from build123d import *

# Parameters (mm, degrees)
EXTRUDE_1_DEPTH          = 3
EXTRUDE_START            = 58
EXTRUDE_2_DEPTH          = 58
EXTRUDE_3_DEPTH          = 0.0001
EXTRUDE_3_DEPTH_BACK     = 6
SKETCH_3_R               = 40
CUT_EXTRUDE_1_DEPTH      = 295.262309003
CUT_EXTRUDE_1_DEPTH_BACK = 295.262309003
EXTRUDE_4_REACH          = 329.042
EXTRUDE_4_END_RADIUS     = 40
SKETCH_5_R               = 28
SKETCH_5_R_2             = 24
RIB_5_REACH              = 296.262
SKETCH_9_WALL_W          = 606.033549296
SKETCH_9_WALL_H          = 6
PATTERN_CIRCULAR_1_COUNT = 4
SKETCH_10_R              = 10
CUT_EXTRUDE_2_DEPTH      = 333.851693714
SKETCH_11_R              = 8
CUT_EXTRUDE_3_DEPTH      = 296.010593044
SKETCH_12_R              = 8
CUT_EXTRUDE_4_DEPTH      = 296.010593044
SKETCH_13_R              = 9.5
CUT_EXTRUDE_5_DEPTH      = 5
SKETCH_14_R              = 1.5
CUT_EXTRUDE_6_DEPTH      = 296.010593044
PATTERN_CIRCULAR_2_COUNT = 6


with BuildPart() as part:
    # Sketch 1 → Extrude 1 (new, symmetric)
    with BuildSketch(Plane(origin=(0, 0, 0), x_dir=(1, 0, 0), z_dir=(0, 1, 0))):
        with BuildLine():
            Line((0, 40), (218, 40))
            ThreePointArc((218, 40), (258, 0), (218, -40))
            Line((218, -40), (0, -40))
            ThreePointArc((0, -40), (-40, 0), (0, 40))
        make_face()
    extrude_1 = extrude(amount=EXTRUDE_1_DEPTH, both=True)

    # Sketch 2 → Extrude 2 (add)
    with BuildSketch(Plane(origin=(0, 3, 0), x_dir=(-1, 0, 0), z_dir=(0, 1, 0)).offset(EXTRUDE_START)):
        with BuildLine():
            Line((-218, -31.8672587), (-218, -40))
            ThreePointArc((-218, -40), (-258, 0), (-218, 40))
            Line((-218, 40), (-218, 31.8672587))
            ThreePointArc((-218, 31.8672587), (-249.8672587, 0), (-218, -31.8672587))
        make_face()
    extrude(amount=-EXTRUDE_2_DEPTH)



with BuildPart() as body_2:
    # Sketch 3 → Extrude 3 (new, two sides: drawn at the far end of the back side and taken through both)
    with BuildSketch(Plane(origin=(282.5, 0, 0), x_dir=(0, 0, -1), z_dir=(1, 0, 0)).offset(-EXTRUDE_3_DEPTH_BACK)):
        with Locations((0, 32)):
            Circle(SKETCH_3_R)
    extrude(amount=EXTRUDE_3_DEPTH + EXTRUDE_3_DEPTH_BACK)

    # Sketch 4 → Cut-Extrude 1 (cut, two sides: drawn at the far end of the back side and taken through both)
    with BuildSketch(Plane.XY.offset(-CUT_EXTRUDE_1_DEPTH_BACK)):
        Polygon((282.5, 835.056567442), (282.5, 76.149376548), (282.5, -15.878690732), (330.214333685, 15.814216416), (962.375669635, 435.709643541), (1731.108568613, 1744.453402873), (1051.232898978, 2143.800326773), align=None)
    extrude(amount=CUT_EXTRUDE_1_DEPTH + CUT_EXTRUDE_1_DEPTH_BACK, mode=Mode.SUBTRACT)


with BuildPart() as part_1:
    add(part.part)

    add(body_2.part)  # Extrude 4 merges body 2
    # Extrude 4: up to this cylinder (the profile starts outside it)
    extrude_4_end = Plane(origin=(218, 32, 0), z_dir=(0, -1, 0)) * Cylinder(EXTRUDE_4_END_RADIUS, 739.084, mode=Mode.PRIVATE)
    # Sketch 5 → Extrude 4 (add, up to the surface)
    with BuildSketch(Plane.ZY.offset(-276.5), mode=Mode.PRIVATE) as extrude_4_sk1:
        with Locations(Location((0, 32, 0), (0, 0, 180))):
            Circle(SKETCH_5_R)
        with Locations(Location((0, 32, 0), (0, 0, 180))):
            Circle(SKETCH_5_R_2, mode=Mode.SUBTRACT)
    extrude_4_tool1 = extrude(extrude_4_sk1.sketch, amount=EXTRUDE_4_REACH, mode=Mode.PRIVATE) - extrude_4_end
    add(extrude_4_tool1.solids().sort_by_distance((276.5, 32, 27.20804))[0])

    # Sketch 9 wall → Rib 5 (add, up to next)
    with BuildSketch(Plane(origin=(269.759419485, 0.166228951, 0), x_dir=(-0.869240691269, 0.49438913888, 0), z_dir=(-0.49438913888, -0.869240691269, 0)), mode=Mode.PRIVATE) as rib_5_sk1:
        Rectangle(SKETCH_9_WALL_W, SKETCH_9_WALL_H)
    rib_5_tool1 = extrude(rib_5_sk1.sketch, amount=-RIB_5_REACH, mode=Mode.PRIVATE) - part_1.part
    rib_5 = rib_5_tool1.solids().sort_by_distance((269.759419485, 0.166228951, 0))[0]
    add(rib_5)

    # Pattern Circular 1: Rib 5 ×4 about axis
    pattern_circular_1_axis = Axis((0, 32, 0), (1, 0, 0))
    for i in range(1, PATTERN_CIRCULAR_1_COUNT):
        add(rib_5.rotate(pattern_circular_1_axis, i * 360 / PATTERN_CIRCULAR_1_COUNT))

    # Mirror 1: Extrude 1 across plane
    add(extrude_1.mirror(Plane.ZX.offset(32)))

    # Sketch 10 → Cut-Extrude 2 (cut, through all)
    with BuildSketch(Plane(origin=(282.5, 0, 0), x_dir=(0, 0, -1), z_dir=(1, 0, 0))):
        with Locations((0, 32)):
            Circle(SKETCH_10_R)
    extrude(amount=-CUT_EXTRUDE_2_DEPTH, mode=Mode.SUBTRACT)

    # Sketch 11 → Cut-Extrude 3 (cut, through all)
    with BuildSketch(Plane(origin=(0, 67, 0), x_dir=(-1, 0, 0), z_dir=(0, 1, 0))):
        with Locations(Location((0, 0, 0), (0, 0, 90))):
            Circle(SKETCH_11_R)
    extrude(amount=-CUT_EXTRUDE_3_DEPTH, mode=Mode.SUBTRACT)

    # Sketch 12 → Cut-Extrude 4 (cut, through all)
    with BuildSketch(Plane(origin=(0, 67, 0), x_dir=(-1, 0, 0), z_dir=(0, 1, 0))):
        with Locations(Location((-72, 0, 0), (0, 0, 90))):
            Circle(SKETCH_12_R)
    extrude(amount=-CUT_EXTRUDE_4_DEPTH, mode=Mode.SUBTRACT)

    # Sketch 13 → Cut-Extrude 5 (cut)
    with BuildSketch(Plane(origin=(0, 3, 0), x_dir=(-1, 0, 0), z_dir=(0, 1, 0))):
        with Locations(Location((-72, 0, 0), (0, 0, 90))):
            Circle(SKETCH_13_R)
        with Locations(Location((0, 0, 0), (0, 0, 90))):
            Circle(SKETCH_13_R)
    cut_extrude_5 = extrude(amount=-CUT_EXTRUDE_5_DEPTH, mode=Mode.SUBTRACT)

    # Mirror 2: Cut-Extrude 5 across plane
    add(cut_extrude_5.mirror(Plane.ZX.offset(32)), mode=Mode.SUBTRACT)

    # Sketch 14 → Cut-Extrude 6 (cut, through all)
    with BuildSketch(Plane(origin=(0, 67, 0), x_dir=(-1, 0, 0), z_dir=(0, 1, 0))):
        with Locations(Location((-41, 0, 0), (0, 0, 90))):
            Circle(SKETCH_14_R)
    cut_extrude_6 = extrude(amount=-CUT_EXTRUDE_6_DEPTH, mode=Mode.SUBTRACT)

    # Pattern Circular 2: Cut-Extrude 6 ×6 about axis
    pattern_circular_2_axis = Axis((72, 0, 0), (0, 1, 0))
    for i in range(1, PATTERN_CIRCULAR_2_COUNT):
        add(cut_extrude_6.rotate(pattern_circular_2_axis, i * 360 / PATTERN_CIRCULAR_2_COUNT), mode=Mode.SUBTRACT)


solid = part_1.part
Geometry check sheet. Reference: the model listing, model coordinates, mm. A direction names the side the tool comes from. Coordinates: 2 decimals unless noted, no trailing zeros. Order: outer loops, then holes, each group sorted by start corner. A loop starts at its lowest first (then second) coordinate and runs counter-clockwise, first axis right, second up. Notation, with made-up numbers: (70, -7.75) -> (90, -7.75) arc R27 ccw to (90, 31.25) -> close; hole circle Ø3 at (-5.5, 72). An arc over 180 degrees is marked (long way). Use a Markdown table: item, result. Add a question column.
1. Cross-section at B-B (z = 20). Enter the section's corners in (x, y).
2. Material ranges on L1, parallel to Y at x = 117, z = 27.5; L2, parallel to X at y = 0.85, z = 0; L3, parallel to X at y = 63.7, z = 0, recorded low to high.
3. Cross-section at D-D (y = 51.5). Enter the section's corners in (x, z), and give its area (3 significant figures).
4. Go/stop test with flat-tipped pins: pin 1 Ø4 at (x, y) = (266.5, 2) entering from +Z; pin 2 Ø24 at (x, z) = (112, -3.5) entering from -Y; pin 3 Ø2.5 at (x, z) = (273, 31.5) entering from -Y; pin 4 Ø1.8 at (x, z) = (56.5, 26.85) entering from -Y. Record where each tip stops, or that it passes through.
5. Set-up check for faces 5 (the face through (269.7, 63.8, 0)), 6 (the face through (276.5, 32.3, -10.3)), 7 (the face through (272, 35, -31)): record each of +Z, -Z, +X, -X, +Y, -Y from which the full face is reachable in a straight line by a thin tool's end or side.
6. Mould release check, pull along X, two halves, no side actions. Record for faces 1 (the face through (218, 32, -36)), 2 (the face through (272, 29, 31)), 3 (the face through (279.46, -7.05, 8.67)), 4 (the face through (-7.81, 66.51, -1.73)): pulls with the +X half, pulls with the -X half, needs draft (parallel to the pull), parting line crosses it, or undercut.
7. Cross-section at C-C (y = 25). Enter the section's corners in (x, z), and give its area (3 significant figures).
8. Cross-section at A-A (x = 145). Enter the section's corners in (y, z), and give its area (3 significant figures).
Filled sheet:
| question | item | result |
|---|---|---|
| 1 | outline | (-34.64, -3) -> (252.64, -3) -> (252.64, 12.4) -> (276.5, 12.4) -> (276.5, -2.64) -> (282.5, -2.64) -> (282.5, 66.64) -> (276.5, 66.64) -> (276.5, 51.6) -> (252.64, 51.6) -> (252.64, 67) -> (-34.64, 67) -> (-34.64, 61) -> (242.81, 61) -> (242.81, 3) -> (-34.64, 3) -> close; hole (252.64, 18.73) -> (276.5, 18.73) -> (276.5, 45.27) -> (252.64, 45.27) -> close |
| 2 | L1 | -3 to 3, 61 to 67 |
| 2 | L2 | -40 to -9.5, 9.5 to 39.5, 42.5 to 62.5, 81.5 to 101.5, 104.5 to 258, 268.56 to 282.5 |
| 2 | L3 | -40 to -9.5, 9.5 to 39.5, 42.5 to 62.5, 81.5 to 101.5, 104.5 to 258, 269.52 to 282.5 |
| 3 | outline | (218, -40) arc R40 ccw to (252.59, -20.09) -> (276.5, -20.09) -> (276.5, -34.92) -> (282.5, -34.92) -> (282.5, 34.92) -> (276.5, 34.92) -> (276.5, 20.09) -> (252.59, 20.09) arc R40 ccw to (218, 40) -> (218, 31.87) arc R31.87 cw to (218, -31.87) -> close; hole (255.47, -13.99) -> (276.5, -13.99) -> (276.5, 13.99) -> (255.47, 13.99) arc R40 cw to start |
| 3 | area | 1,610 mm2 |
| 4 | pin 1 | z = 3 |
| 4 | pin 2 | y = -3 |
| 4 | pin 3 | y = 29 |
| 4 | pin 4 | through |
| 5 | face 5 | +Z, -Z, +Y |
| 5 | face 6 | none |
| 5 | face 7 | -Z, +Y |
| 6 | face 1 | pulls with the -X half |
| 6 | face 2 | undercut |
| 6 | face 3 | needs draft |
| 6 | face 4 | undercut |
| 7 | outline | (218, -40) arc R40 ccw to (247.41, -27.11) -> (276.5, -27.11) -> (276.5, -39.38) -> (282.5, -39.38) -> (282.5, -7.14) -> (276.5, -7.14) -> (276.5, -22.96) -> (250.76, -22.96) arc R40 ccw to (257.36, -7.14) -> (249.06, -7.14) arc R31.87 cw to (218, -31.87) -> close; (218, 31.87) arc R31.87 cw to (249.06, 7.14) -> (257.36, 7.14) arc R40 ccw to (250.76, 22.96) -> (276.5, 22.96) -> (276.5, 7.14) -> (282.5, 7.14) -> (282.5, 39.38) -> (276.5, 39.38) -> (276.5, 27.11) -> (247.41, 27.11) arc R40 ccw to (218, 40) -> close |
| 7 | area | 1,420 mm2 |
| 8 | outline | (-3, -40) -> (3, -40) -> (3, 40) -> (-3, 40) -> close; (61, -40) -> (67, -40) -> (67, 40) -> (61, 40) -> close |
| 8 | area | 960 mm2 |
